from build123d import *

# Parameters (mm, degrees)
F0_R     = 11
F1_DEPTH = 3.5
F2_R     = 2
F3_R     = 2
F4_DEPTH = 1.5


with BuildPart() as f1:
    # F0 (on Top) → F1 (new body, symmetric)
    with BuildSketch(Plane.XY):
        with BuildLine():
            ThreePointArc((-0.8285496132, 17.1446015607), (-1.0500524725, 15.314704152), (-2.5690728422, 14.2705944071))
            ThreePointArc((-2.5690728422, 14.2705944071), (-6.985549163, 12.7063804009), (-10.6726700751, 9.8155037297))
            Line((-10.6726700751, 9.8155037297), (-40.2240356418, -22.3165175753))
            ThreePointArc((-40.2240356418, -22.3165175753), (-37.447016124, -26.7155569548), (-34.1910537852, -30.7729075821))
            Line((-34.1910537852, -30.7729075821), (-14.4333856827, -9.2898457936))
            ThreePointArc((-14.4333856827, -9.2898457936), (-12.7378966108, -8.5667241925), (-11.0741608625, -9.3601795491))
            ThreePointArc((-11.0741608625, -9.3601795491), (-7.5112736358, -12.4028532349), (-3.1641405433, -14.1505552761))
            Line((-3.1641405433, -14.1505552761), (39.4386889651, -23.6767779209))
            ThreePointArc((39.4386889651, -23.6767779209), (41.8598590611, -19.0722887819), (43.745646607, -14.2238673691))
            Line((43.745646607, -14.2238673691), (15.2619352959, -7.8547557671))
            ThreePointArc((15.2619352959, -7.8547557671), (13.7879490833, -6.7479799595), (13.6432337047, -4.910414858))
            ThreePointArc((13.6432337047, -4.910414858), (14.4968227988, -0.3035271659), (13.8368106184, 4.3350515464))
            Line((13.8368106184, 4.3350515464), (0.7853466767, 45.9932954962))
            ThreePointArc((0.7853466767, 45.9932954962), (-4.4128429371, 45.7878457368), (-9.5545928219, 44.9967749512))
            Line((-9.5545928219, 44.9967749512), (-0.8285496132, 17.1446015607))
        make_face()
        Circle(F0_R, mode=Mode.SUBTRACT)
        with BuildLine():
            Line((-10.3051834804, 47.3925436481), (-9.5545928219, 44.9967749512))
            ThreePointArc((-9.5545928219, 44.9967749512), (-4.4128429371, 45.7878457368), (0.7853466767, 45.9932954962))
            Line((0.7853466767, 45.9932954962), (0, 48.5))
            ThreePointArc((0, 48.5), (-5.1822597903, 48.2223411239), (-10.3051834804, 47.3925436481))
        make_face()
        with BuildLine():
            ThreePointArc((43.745646607, -14.2238673691), (41.8598590611, -19.0722887819), (39.4386889651, -23.6767779209))
            Line((39.4386889651, -23.6767779209), (42.0022320835, -24.25))
            ThreePointArc((42.0022320835, -24.25), (44.3529023384, -19.6232019345), (46.1957384894, -14.7717211394))
            Line((46.1957384894, -14.7717211394), (43.745646607, -14.2238673691))
        make_face()
        with BuildLine():
            ThreePointArc((-34.1910537852, -30.7729075821), (-37.447016124, -26.7155569548), (-40.2240356418, -22.3165175753))
            Line((-40.2240356418, -22.3165175753), (-42.0022320835, -24.25))
            ThreePointArc((-42.0022320835, -24.25), (-39.1706425481, -28.5991391893), (-35.890555009, -32.6208225087))
            Line((-35.890555009, -32.6208225087), (-34.1910537852, -30.7729075821))
        make_face()
    extrude(amount=F1_DEPTH, both=True)

    # F2
    f2_edges = [f1.edges().sort_by_distance(p)[0] for p in [
        (-26.337451, -7.217248, 3.5),
        (-6.985549, 12.70638, 3.5),
        (-1.050052, 15.314704, 3.5),
        (-5.566867, 32.268573, 3.5),
        (6.918405, 26.417526, 3.5),
        (14.496823, -0.303527, 3.5),
        (13.787949, -6.74798, 3.5),
        (30.728837, -11.313238, 3.5),
        (19.419046, -19.200278, 3.5),
        (-7.511274, -12.402853, 3.5),
        (-12.737897, -8.566724, 3.5),
        (-25.16197, -20.955334, 3.5),
    ]]
    fillet(f2_edges, radius=F2_R)

    # F3
    f3_edges = [f1.edges().sort_by_distance(p)[0] for p in [
        (-26.337451, -7.217248, -3.5),
        (-6.985549, 12.70638, -3.5),
        (-1.050052, 15.314704, -3.5),
        (-5.566867, 32.268573, -3.5),
        (6.918405, 26.417526, -3.5),
        (14.496823, -0.303527, -3.5),
        (13.787949, -6.74798, -3.5),
        (30.728837, -11.313238, -3.5),
        (19.419046, -19.200278, -3.5),
        (-7.511274, -12.402853, -3.5),
        (-12.737897, -8.566724, -3.5),
        (-25.16197, -20.955334, -3.5),
    ]]
    fillet(f3_edges, radius=F3_R)


with BuildPart() as f4:
    # F0 (on Top) → F4 (new body, symmetric)
    with BuildSketch(Plane.XY):
        with BuildLine():
            Line((-10.3051834804, 47.3925436481), (-9.5545928219, 44.9967749512))
            ThreePointArc((-9.5545928219, 44.9967749512), (-4.4128429371, 45.7878457368), (0.7853466767, 45.9932954962))
            Line((0.7853466767, 45.9932954962), (0, 48.5))
            ThreePointArc((0, 48.5), (-5.1822597903, 48.2223411239), (-10.3051834804, 47.3925436481))
        make_face()
        with BuildLine():
            Line((-42.0022320835, -24.25), (-40.2240356418, -22.3165175753))
            ThreePointArc((-40.2240356418, -22.3165175753), (-41.8598590611, 19.0722887819), (-9.5545928219, 44.9967749512))
            Line((-9.5545928219, 44.9967749512), (-10.3051834804, 47.3925436481))
            ThreePointArc((-10.3051834804, 47.3925436481), (-44.3529023384, 19.6232019345), (-42.0022320835, -24.25))
        make_face()
        with BuildLine():
            ThreePointArc((-34.1910537852, -30.7729075821), (-37.447016124, -26.7155569548), (-40.2240356418, -22.3165175753))
            Line((-40.2240356418, -22.3165175753), (-42.0022320835, -24.25))
            ThreePointArc((-42.0022320835, -24.25), (-39.1706425481, -28.5991391893), (-35.890555009, -32.6208225087))
            Line((-35.890555009, -32.6208225087), (-34.1910537852, -30.7729075821))
        make_face()
        with BuildLine():
            ThreePointArc((39.4386889651, -23.6767779209), (4.4128429371, -45.7878457368), (-34.1910537852, -30.7729075821))
            Line((-34.1910537852, -30.7729075821), (-35.890555009, -32.6208225087))
            ThreePointArc((-35.890555009, -32.6208225087), (5.1822597903, -48.2223411239), (42.0022320835, -24.25))
            Line((42.0022320835, -24.25), (39.4386889651, -23.6767779209))
        make_face()
        with BuildLine():
            ThreePointArc((43.745646607, -14.2238673691), (41.8598590611, -19.0722887819), (39.4386889651, -23.6767779209))
            Line((39.4386889651, -23.6767779209), (42.0022320835, -24.25))
            ThreePointArc((42.0022320835, -24.25), (44.3529023384, -19.6232019345), (46.1957384894, -14.7717211394))
            Line((46.1957384894, -14.7717211394), (43.745646607, -14.2238673691))
        make_face()
        with BuildLine():
            Line((0, 48.5), (0.7853466767, 45.9932954962))
            ThreePointArc((0.7853466767, 45.9932954962), (32.8033988112, 32.2480546147), (46, 0))
            ThreePointArc((46, 0), (45.4329161728, -7.2007033016), (43.745646607, -14.2238673691))
            Line((43.745646607, -14.2238673691), (46.1957384894, -14.7717211394))
            ThreePointArc((46.1957384894, -14.7717211394), (47.9204722261, -7.4751817123), (48.5, 0))
            ThreePointArc((48.5, 0), (34.2946788875, 34.2946788875), (0, 48.5))
        make_face()
    extrude(amount=F4_DEPTH, both=True)


with BuildPart() as f1_1:
    add(f1.part)

    # F5: cut F4
    add(f4.part, mode=Mode.SUBTRACT)


solid = f1_1.part
The model under review builds one solid part; all positions refer to its coordinate system, in mm. A direction names the side the tool comes from. Give positions to 0.01 mm unless a question says otherwise; leave off trailing zeros.
1. Draft analysis for pull direction Y (two halves, no side actions). For faces 6 (the cylindrical face through (-1.036, 15.338, 0.021)), 7 (the cylindrical face through (-26.31, -8.08, -2.93)), 8 (the flat face through (-11, -3, -3.5)), 9 (the flat face through (-5.253, 31.266, 0.021)), state which applies: +Y half, -Y half, draft (parallel to the pull), parting line (faces both ways), or undercut.
2. Wall thickness on L1, parallel to Y at x = 0, z = 0.75; L2, parallel to Y at x = 18, z = -1.5; L3, parallel to Y at x = 24, z = 0.25: over which ranges is each line inside the solid? List them lowest first.
3. Tool access review of faces 1 (the flat face through (-24.45, -20.18, 0.02)), 2 (the flat face through (-5, 47, 1.5)), 3 (the cylindrical face through (-6.928, 12.738, 0.021)), 4 (the flat face through (-38, -27, -1.5)), 5 (the flat face through (43, -19, 1.5)): name each direction out of +Z, -Z, +X, -X, +Y, -Y from which nothing blocks a thin tool from reaching the whole face with its end or side.
Worked answers:
1. face 6: undercut
1. face 7: +Y half
1. face 8: draft
1. face 9: undercut
2. L1: y = -14.86 to -11, 11 to 46
2. L2: y = -18.88 to -8.47
2. L3: y = -20.22 to -9.81
3. face 1: +Z, -Z, -Y
3. face 2: -X, +Y
3. face 3: +Z, -Z, -X
3. face 4: -X, -Y
3. face 5: +X, -Y
